Part print with two shaded views. Sizes in mm from the minimum x, y, z corner. A direction names the side the tool comes from. Give positions to 0.01 mm unless a question says otherwise; leave off trailing zeros. Loops run counter-clockwise (first coordinate to the right, second up) from the corner with the lowest first, then second, coordinate; pieces in that order, holes last. Notation, with made-up numbers: M 20.5,20 L 33.5,20 A19 ccw 33.5,56 Z; hole C 43.5,66 d7. An arc over 180 degrees is marked long. Answer as a JSON object with one key per item and string values. Group by question number.
1. 3-axis set-ups, long thin cutter, end or side, ignore diameter. For the marked faces 4, 5 and 6: which of +Z, -Z, +X, -X, +Y, -Y reach the whole face in a straight line?
2. Slice it at A-A (y = 54). List the corners of the cut face in (x, z).
3. Drill centre lines: line 1 along Z through (x, y) = (41.5, 13.5); line 2 along X through (y, z) = (44.5, 16.75); line 3 along Y through (x, z) = (53.5, 5). Where is each one in solid material? Low to high. Write a range as [from, to].
4. Slice it at B-B (z = 13.75). List the corners of the cut face in (x, y).
5. Slice it at D-D (z = 23.25). List the corners of the cut face in (x, y).
6. Slice it at C-C (x = 45). List the corners of the cut face in (y, z) (1 decimal).
7. Mould opens along X. For the marked faces 1, 2 and 3 say: released by +X, released by -X, zero draft, split by the parting line, or undercut.
8. Drop flat-ended pins along their axis: pin 1 Ø1.5 at (x, z) = (44.5, 16) entering from +Y (1 decimal); pin 2 Ø4 at (x, z) = (3, 9) entering from +Y; pin 3 Ø4.5 at (x, z) = (8, 10.5) entering from +Y. Give the stop position or say it passes through.
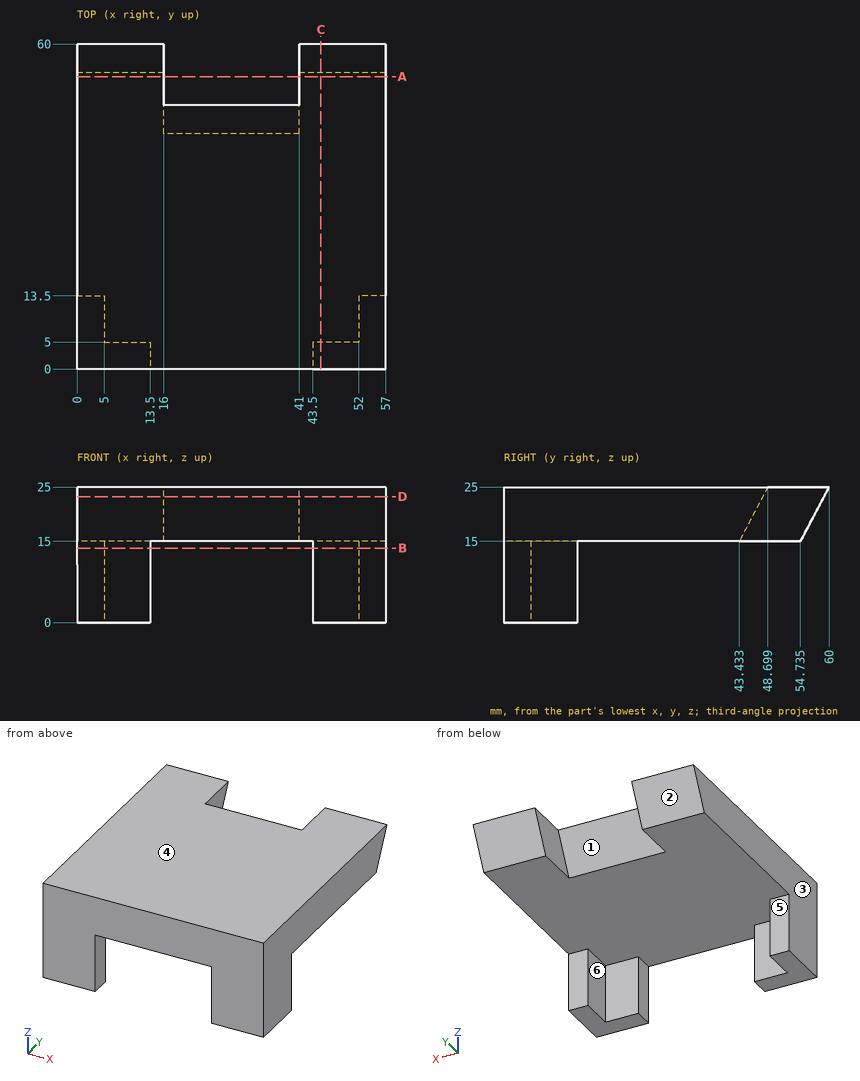
Established:
{
 "1": {"face 4": "+Z, +X, -X, +Y, -Y", "face 5": "-Z, +X, -X, +Y", "face 6": "-Z, +Y"},
 "2": {"outline": "M 0,15 L 16,15 L 16,25 L 0,25 Z; M 41,15 L 57,15 L 57,25 L 41,25 Z"},
 "3": {"line 1": "z = [15, 25]", "line 2": "x = [0, 16], [41, 57]", "line 3": "y = [0, 13.5]"},
 "4": {"outline": "M 0,0 L 13.5,0 L 13.5,5 L 5,5 L 5,13.5 L 0,13.5 Z; M 43.5,0 L 57,0 L 57,13.5 L 52,13.5 L 52,5 L 43.5,5 Z"},
 "5": {"outline": "M 0,0 L 57,0 L 57,59.08 L 41,59.08 L 41,47.78 L 16,47.78 L 16,59.08 L 0,59.08 Z"},
 "6": {"outline": "M 0,0 L 5,0 L 5,15 L 54.7,15 L 60,25 L 0,25 Z"},
 "7": {"face 1": "undercut", "face 2": "zero draft", "face 3": "released by -X"},
 "8": {"pin 1": "stops at y = 55.7", "pin 2": "stops at y = 13.5", "pin 3": "stops at y = 5"}
}
